```python
from build123d import *

# Parameters (mm, degrees)
SKETCH1_W             = 25
SKETCH1_H             = 90
BOSS_EXTRUDE1_DEPTH   = 13
SKETCH2_W             = 20
SKETCH2_H             = 70
CUT_EXTRUDE1_DEPTH    = 23
FILLET1_R             = 5
M4X0_7_TAPPED_HOLE1_D = 3.3


with BuildPart() as part:
    # Sketch1 → Boss-Extrude1 (new body)
    with BuildSketch(Plane.XY):
        Rectangle(SKETCH1_W, SKETCH1_H)
    extrude(amount=BOSS_EXTRUDE1_DEPTH)

    # Sketch2 → Cut-Extrude1 (cut)
    with BuildSketch(Plane.XY.offset(13)):
        Rectangle(SKETCH2_W, SKETCH2_H)
    extrude(amount=-CUT_EXTRUDE1_DEPTH, mode=Mode.SUBTRACT)

    # Fillet1
    fillet1_edges = [part.edges().sort_by_distance(p)[0] for p in [
        (10, 35, 6.5),
        (10, -35, 6.5),
        (-10, -35, 6.5),
        (-10, 35, 6.5),
    ]]
    fillet(fillet1_edges, radius=FILLET1_R)

    # M4x0.7 Tapped Hole1 (through all)
    with Locations(Plane(origin=(0, -45, 0), x_dir=(-1, 0, 0), z_dir=(0, -1, 0))):
        with Locations((-5, -5), (5, -5)):
            Hole(M4X0_7_TAPPED_HOLE1_D / 2)


solid = part.part
```
Geometry check sheet. Reference: the model listing, model coordinates, mm. A direction names the side the tool comes from. Give positions to 0.01 mm unless a question says otherwise; leave off trailing zeros. Write each loop counter-clockwise with the first axis right and the second up, starting at its lowest first coordinate (ties: lowest second). Pieces come first, ordered by that corner, then holes. Notation, with made-up numbers: (78.5, 35) - (126.5, 35) arc R20 cw to (126.5, 57) - close; hole circle Ø3 at (55, -17). An arc over 180 degrees is marked (long way). Use a Markdown table: item, result.
Q1. Section check D-D, the plane z = 5. Enter the section's corners in (x, y), then the cut area to 3 significant figures.
Computed:
| item | result |
|---|---|
| outline | (-12.5, -45) - (-6.65, -45) - (-6.65, -34.72) arc R5 cw to (-10, -30) - (-10, 30) arc R5 cw to (-6.65, 34.72) - (-6.65, 45) - (-12.5, 45) - close; (-3.35, -45) - (3.35, -45) - (3.35, -35) - (-3.35, -35) - close; (-3.35, 35) - (3.35, 35) - (3.35, 45) - (-3.35, 45) - close; (6.65, -45) - (12.5, -45) - (12.5, 45) - (6.65, 45) - (6.65, 34.72) arc R5 cw to (10, 30) - (10, -30) arc R5 cw to (6.65, -34.72) - close |
| area | 739 mm² |
Q2. Section check C-C, the plane z = 10.25. Enter the section's corners in (x, y).
Computed:
| item | result |
|---|---|
| outline | (-12.5, -45) - (12.5, -45) - (12.5, 45) - (-12.5, 45) - close; hole (-10, -30) arc R5 ccw to (-5, -35) - (5, -35) arc R5 ccw to (10, -30) - (10, 30) arc R5 ccw to (5, 35) - (-5, 35) arc R5 ccw to (-10, 30) - close |
Q3. Go/stop test with a flat-tipped pin: P1, Ø3, axis at x = -5, z = 5, coming from the +Y side. Record where the tip stops, or that it passes through.
Computed:
| item | result |
|---|---|
| P1 | passes through |
Q4. Section check A-A, the plane y = 22.5. Enter the section's corners in (x, z), then the cut area to 3 significant figures.
Computed:
| item | result |
|---|---|
| outline | (-12.5, 0) - (-10, 0) - (-10, 13) - (-12.5, 13) - close; (10, 0) - (12.5, 0) - (12.5, 13) - (10, 13) - close |
| area | 65.0 mm² |
Q5. Draft check along Z on faces 3 (the face through (0, 35, 7)), 4 (the face through (-11, 1, 0)), 5 (the face through (3.35, -39.79, 4.93)). Enter one of: pulls with the +Z half, pulls with the -Z half, needs draft (parallel to the pull), parting line crosses it, or undercut.
Computed:
| item | result |
|---|---|
| face 3 | needs draft |
| face 4 | pulls with the -Z half |
| face 5 | undercut |
Q6. Thickness scan on L1, parallel to X at y = 39.5, z = 5; L2, parallel to X at y = 24, z = 10.75; L3, parallel to Y at x = 2, z = 6.5. Record the ranges inside material, lowest first. Write a range as [from, to].
Computed:
| item | result |
|---|---|
| L1 | x = [-12.5, -6.65], [-3.35, 3.35], [6.65, 12.5] |
| L2 | x = [-12.5, -10], [10, 12.5] |
| L3 | y = [-45, -35], [35, 45] |
Q7. Section check B-B, the plane x = -0.5. Enter the section's corners in (y, z).
Computed:
| item | result |
|---|---|
| outline | (-45, 0) - (-35, 0) - (-35, 13) - (-45, 13) - close; (35, 0) - (45, 0) - (45, 13) - (35, 13) - close |
Q8. Set-up check for faces 1 (the face through (12.5, -1, 6)), 2 (the face through (10, 0, 7)): record each of +Z, -Z, +X, -X, +Y, -Y from which the full face is reachable in a straight line by a thin tool's end or side.
Computed:
| item | result |
|---|---|
| face 1 | +Z, -Z, +X, +Y, -Y |
| face 2 | +Z, -Z |
